CAD build for the part. Positions are in the model's coordinates, mm. Give positions to 0.01 mm unless a question says otherwise; leave off trailing zeros. Write each loop counter-clockwise with the first axis right and the second up, starting at its lowest first coordinate (ties: lowest second). Pieces come first, ordered by that corner, then holes. Notation, with made-up numbers: (-18, -14) - (24, -14) arc R13 ccw to (24, -9) - close; hole circle Ø9 at (59.5, 24). An arc over 180 degrees is marked (long way). Put each result on its own line as item: value. Start each with the question number.
1. Mould opens along Y. For faces 1 (the flat face through (0, -43.02, 6)), 2 (the flat face through (10, -1, 6)), 3 (the cylindrical face through (-1.072, -3.405, 5.916)) say: +Y half, -Y half, draft (parallel to the pull), parting line (faces both ways), or undercut.
2. Cut at B-B on y = 0. List the corners of the cut face in (x, z).
3. Cut at A-A on x = 0. List the corners of the cut face in (y, z), and give its area (3 significant figures).
4. Wall check: line 1 (Y direction, x = 0, z = 5.25); line 2 (X direction, y = -20.32, z = 6.5); line 3 (Y direction, x = -1.5, z = 6). Give the ranges that are in metal, low to high.
5. Drop a flat-ended pin along its axis: pin 1 (5 mm diameter, centred on x = 8, y = -18.5, fed in from -Z). Give the stop position or say it passes through.
6. Cut at D-D on y = -20.32. List the corners of the cut face in (x, z).
7. Cut at C-C on z = 6.5. List the corners of the cut face in (x, y).
Autodesk Inventor part; units mm, degrees
ref_plane "YZ Plane" through (0, 0, 0) normal (1, 0, 0) x (0, 1, 0)
ref_plane "XZ Plane" through (0, 0, 0) normal (0, 1, 0) x (-1, 0, 0)
ref_plane "XY Plane" through (0, 0, 0) normal (0, 0, 1) x (1, 0, 0)
sketch "Sketch1" plane through (0, 0, 0) normal (0, 0, 1) x (1, 0, 0)
  line L0 (-10, -43.02) -> (10, -43.02)
  line L1 (10, -43.02) -> (10, 43.02)
  line L2 (10, 43.02) -> (-10, 43.02)
  line L3 (-10, 43.02) -> (-10, -43.02)
  line L4 (-10, -43.02) -> (10, 43.02) construction
  line L5 (10, -43.02) -> (-10, 43.02) construction
  point P0 (0, 0)
  dimension "d0" = 20
  dimension "d1" = 86.04
extrude "Extrusion1" add sketch "Sketch1" along normal blind 12
sketch "Sketch2" plane through (0, 0, 12) normal (0, 0, 1) x (1, 0, 0)
  point P0 (0, 0)
  point P1 (0, 0)
  point P2 (0, 30.32)
  point P3 (0, -30.32)
  dimension "d4" = 30.32
  dimension "d5" = 30.32
hole "Hole1" at (0, 0, 12) at (0, 30.32, 12) at (0, -30.32, 12) direction (0, 0, -1) diameter 7.14 end through all
sketch "Sketch3" plane through (0, 0, 12) normal (0, 0, 1) x (1, 0, 0)
  circle A0 centre (0, 0) radius 3.57
  point P0 (0, 20.32)
  point P1 (0, -20.32)
  dimension "d13" = 20.32
  dimension "d14" = 20.32
hole "Hole2" at (0, 20.32, 12) at (0, -20.32, 12) direction (0, 0, -1) diameter 4.134 end through all
fillet "Fillet1" radius 3.36 4 edges at (10, 43.02, 6) (-10, 43.02, 6) (10, -43.02, 6) (-10, -43.02, 6)
properties part number "VSlot Spacer Block" material "Aluminum 6061"
Report:
1. face 1: -Y half
1. face 2: draft
1. face 3: undercut
2. outline: (-10, 0) - (-3.57, 0) - (-3.57, 12) - (-10, 12) - close; (3.57, 0) - (10, 0) - (10, 12) - (3.57, 12) - close
3. outline: (-43.02, 0) - (-33.89, 0) - (-33.89, 12) - (-43.02, 12) - close; (-26.75, 0) - (-22.39, 0) - (-22.39, 12) - (-26.75, 12) - close; (-18.25, 0) - (-3.57, 0) - (-3.57, 12) - (-18.25, 12) - close; (3.57, 0) - (18.25, 0) - (18.25, 12) - (3.57, 12) - close; (22.39, 0) - (26.75, 0) - (26.75, 12) - (22.39, 12) - close; (33.89, 0) - (43.02, 0) - (43.02, 12) - (33.89, 12) - close
3. area: 676 mm²
4. line 1: y = -43.02 to -33.89, -26.75 to -22.39, -18.25 to -3.57, 3.57 to 18.25, 22.39 to 26.75, 33.89 to 43.02
4. line 2: x = -10 to -2.07, 2.07 to 10
4. line 3: y = -43.02 to -33.56, -27.08 to -21.74, -18.9 to -3.24, 3.24 to 18.9, 21.74 to 27.08, 33.56 to 43.02
5. pin 1: stops at z = 0
6. outline: (-10, 0) - (-2.07, 0) - (-2.07, 12) - (-10, 12) - close; (2.07, 0) - (10, 0) - (10, 12) - (2.07, 12) - close
7. outline: (-10, -39.66) arc R3.36 ccw to (-6.64, -43.02) - (6.64, -43.02) arc R3.36 ccw to (10, -39.66) - (10, 39.66) arc R3.36 ccw to (6.64, 43.02) - (-6.64, 43.02) arc R3.36 ccw to (-10, 39.66) - close; hole circle Ø7.14 at (0, -30.32); hole circle Ø7.14 at (0, 0); hole circle Ø7.14 at (0, 30.32); hole circle Ø4.13 at (0, -20.32); hole circle Ø4.13 at (0, 20.32)
